from build123d import *

# Parameters (mm, degrees)
SKETCH2_R           = 13.5
SKETCH2_R_2         = 6
SKETCH2_R_3         = 0.5
BOSS_EXTRUDE2_DEPTH = 2
BOSS_EXTRUDE3_DEPTH = 2.5


with BuildPart() as part:
    # Sketch2 → Boss-Extrude2 (new, symmetric)
    with BuildSketch(Plane.XY):
        Circle(SKETCH2_R)
        Circle(SKETCH2_R_2, mode=Mode.SUBTRACT)
        with Locations((8.443747687, 4.875)):
            Circle(SKETCH2_R_3, mode=Mode.SUBTRACT)
        with Locations((0, -9.75)):
            Circle(SKETCH2_R_3, mode=Mode.SUBTRACT)
        with Locations((-8.443747687, 4.875)):
            Circle(SKETCH2_R_3, mode=Mode.SUBTRACT)
    extrude(amount=BOSS_EXTRUDE2_DEPTH, both=True)

    # Sketch3 → Boss-Extrude3 (add, symmetric)
    with BuildSketch(Plane.XY):
        with BuildLine():
            Line((7.632450055, -2.530208719), (6.007450055, -5.344791281))
            ThreePointArc((6.007450055, -5.344791281), (5.982474949, -5.534496042), (6.098956406, -5.686297632))
            Line((6.098956406, -5.686297632), (8.913538968, -7.311297632))
            ThreePointArc((8.913538968, -7.311297632), (9.103243729, -7.336272738), (9.255045319, -7.219791281))
            Line((9.255045319, -7.219791281), (10.880045319, -4.405208719))
            ThreePointArc((10.880045319, -4.405208719), (10.905020425, -4.215503958), (10.788538968, -4.063702368))
            Line((10.788538968, -4.063702368), (7.973956406, -2.438702368))
            ThreePointArc((7.973956406, -2.438702368), (7.784251644, -2.413727262), (7.632450055, -2.530208719))
        make_face()
        with BuildLine():
            Line((-1.375, 7.875), (1.375, 7.875))
            ThreePointArc((1.375, 7.875), (1.728553391, 8.021446609), (1.875, 8.375))
            Line((1.875, 8.375), (1.875, 11.125))
            ThreePointArc((1.875, 11.125), (1.728553391, 11.478553391), (1.375, 11.625))
            Line((1.375, 11.625), (-1.375, 11.625))
            ThreePointArc((-1.375, 11.625), (-1.728553391, 11.478553391), (-1.875, 11.125))
            Line((-1.875, 11.125), (-1.875, 8.375))
            ThreePointArc((-1.875, 8.375), (-1.728553391, 8.021446609), (-1.375, 7.875))
        make_face()
        with BuildLine():
            Line((-6.007450055, -5.344791281), (-7.632450055, -2.530208719))
            ThreePointArc((-7.632450055, -2.530208719), (-7.784251644, -2.413727262), (-7.973956406, -2.438702368))
            Line((-7.973956406, -2.438702368), (-10.788538968, -4.063702368))
            ThreePointArc((-10.788538968, -4.063702368), (-10.905020425, -4.215503958), (-10.880045319, -4.405208719))
            Line((-10.880045319, -4.405208719), (-9.255045319, -7.219791281))
            ThreePointArc((-9.255045319, -7.219791281), (-9.103243729, -7.336272738), (-8.913538968, -7.311297632))
            Line((-8.913538968, -7.311297632), (-6.098956406, -5.686297632))
            ThreePointArc((-6.098956406, -5.686297632), (-5.982474949, -5.534496042), (-6.007450055, -5.344791281))
        make_face()
    extrude(amount=BOSS_EXTRUDE3_DEPTH, both=True)


solid = part.part
Could you check a few things on this model? Use its own coordinates, in mm. A direction names the side the tool comes from. Round coordinates to 2 decimals unless told otherwise and drop trailing zeros. Write each loop counter-clockwise with the first axis right and the second up, starting at its lowest first coordinate (ties: lowest second). Pieces come first, ordered by that corner, then holes. Notation, with made-up numbers: (-27.75, 87) - (-17.75, 87) arc R22 cw to (-17.75, 117) - close; hole circle Ø6 at (85, 44.5). An arc over 180 degrees is marked (long way). Put each result on its own line as item: value. Start each with the question number.
(1) Thinking about a two-plate mould opening in Y: for faces 5 (the flat face through (-6.809, -3.957, 2.254)), 6 (the cylindrical face through (-8.943, 4.897, -0.028)), 7 (the cylindrical face through (-2.93, -13.18, 0.03)), 8 (the cylindrical face through (8.075, 5.213, -0.028)), which applies, released by +Y, released by -Y, zero draft, split by the parting line, or undercut?
(2) I need wall thicknesses on probe 1 along Y at (x, z) = (0, 0.35); probe 2 along Z at (x, y) = (-3.75, -5); probe 3 along X at (y, z) = (2.5, 0.6). Which ranges of each line are inside material? Lowest first, please.
(3) For faces 1 (the flat face through (-10.08, -5.79, -2.25)), 2 (the flat face through (7.49, -6.49, 2.25)), 3 (the flat face through (9.4, -3.26, 2.25)), 4 (the flat face through (6, -3, 2)), which set-ups out of +Z, -Z, +X, -X, +Y, -Y let a thin tool reach every point of the face, with its end or its side?
(4) I want a section at D-D, the plane z = -0.05. Please give me the cut outline in (x, y) (3 decimals).
(5) I want a section at C-C, the plane x = 5.5. Please give me the cut outline in (y, z).
(6) I want a section at B-B, the plane x = 0. Please give me the cut outline in (y, z) (3 decimals), plus the area to 4 significant figures.
(7) I want a section at A-A, the plane y = 0. Please give me the cut outline in (x, z).
(8) Will these pins go through, and if not, where does the flat tip stop? pin 1 (2 mm diameter, centred on x = 1.5, z = -1.5, fed in from +Y); pin 2 (0.6 mm diameter, centred on y = 10.5, z = 2, fed in from +X); pin 3 (2 mm diameter, centred on x = -5.5, z = 1.5, fed in from +Y).
Here are the results:
1. face 5: released by +Y
1. face 6: undercut
1. face 7: split by the parting line
1. face 8: undercut
2. probe 1: y = -13.5 to -10.25, -9.25 to -6, 6 to 13.5
2. probe 2: z = -2 to 2
2. probe 3: x = -13.27 to -5.45, 5.45 to 13.27
3. face 1: -Z, -X, -Y
3. face 2: +Z, -Y
3. face 3: +Z, +X, +Y
3. face 4: +Z
4. outline: circle Ø27 at (0, 0); hole circle Ø1 at (-8.444, 4.875); hole circle Ø12 at (0, 0); hole circle Ø1 at (0, -9.75); hole circle Ø1 at (8.444, 4.875)
5. outline: (-12.33, -2) - (-2.4, -2) - (-2.4, 2) - (-12.33, 2) - close; (2.4, -2) - (12.33, -2) - (12.33, 2) - (2.4, 2) - close
6. outline: (-13.5, -2) - (-10.25, -2) - (-10.25, 2) - (-13.5, 2) - close; (-9.25, -2) - (-6, -2) - (-6, 2) - (-9.25, 2) - close; (6, -2) - (7.875, -2) - (7.875, -2.5) - (11.625, -2.5) - (11.625, -2) - (13.5, -2) - (13.5, 2) - (11.625, 2) - (11.625, 2.5) - (7.875, 2.5) - (7.875, 2) - (6, 2) - close
6. area: 59.75 mm^2
7. outline: (-13.5, -2) - (-6, -2) - (-6, 2) - (-13.5, 2) - close; (6, -2) - (13.5, -2) - (13.5, 2) - (6, 2) - close
8. pin 1: stops at y = 13.49
8. pin 2: stops at x = 8.84
8. pin 3: stops at y = 12.73
